from build123d import *

# Parameters (mm, degrees)
F0_W        = 40
F0_H        = 155
F1_DEPTH    = 3
F2_W        = 12.5
F2_H        = 13
F3_DEPTH    = 3
F4_R        = 8
F5_T1_DEPTH = 3
F6_R        = 1
F7_DEPTH    = 3
F8_DEPTH    = 15.3


# Not quite as in the source:
# - a fillet or chamfer that OpenCascade refuses, or shapes differently, is made with other operations: its cross-section is extruded or revolved along the edge and cut away or added


with BuildPart() as f1:
    # F0 (on Top) → F1 (new body)
    with BuildSketch(Plane.XY):
        Rectangle(F0_W, F0_H)
    extrude(amount=F1_DEPTH)

    # F2 (on face) → F3 (cut, through all)
    with BuildSketch(Plane.XY.offset(3)):
        with Locations((-13.75, -51)):
            Rectangle(F2_W, F2_H)
        with Locations((13.75, -51)):
            Rectangle(F2_W, F2_H)
    extrude(amount=-F3_DEPTH, mode=Mode.SUBTRACT)

    # F4
    f4_edges = [f1.edges().sort_by_distance(p)[0] for p in [
        (-20, -44.5, 1.5),
        (20, -44.5, 1.5),
        (20, -57.5, 1.5),
        (-20, -57.5, 1.5),
        (-20, -77.5, 1.5),
        (20, -77.5, 1.5),
        (-20, 77.5, 1.5),
        (20, 77.5, 1.5),
    ]]
    fillet(f4_edges, radius=F4_R)

    # F5: fillet of radius 7 on 4 edges, made by hand

    # F5_s2 → F5_t1 (join)
    with BuildSketch(Plane.XY):
        with BuildLine():
            ThreePointArc((-13.3333333333, -44.3881063775), (-9.1536616892, -46.7717188872), (-7.5, -51.2901994578))
            Line((-7.5, -51.2901994578), (-6.8, -51.2901994578))
            Line((-6.8, -51.2901994578), (-6.8, -44.5))
            Line((-6.8, -44.5), (-7.5, -43.8))
            ThreePointArc((-7.5, -43.8), (-12, -43.8), (-13.2166666667, -43.6978970694))
            Line((-13.2166666667, -43.6978970694), (-13.3333333333, -44.3881063775))
        make_face()
        with BuildLine():
            ThreePointArc((-7.5, -50.7098005422), (-9.1536616892, -55.2282811128), (-13.3333333333, -57.6118936225))
            Line((-13.3333333333, -57.6118936225), (-13.2166666667, -58.3021029306))
            ThreePointArc((-13.2166666667, -58.3021029306), (-12, -58.2), (-7.5, -58.2))
            Line((-7.5, -58.2), (-6.8, -57.5))
            Line((-6.8, -57.5), (-6.8, -50.7098005422))
            Line((-6.8, -50.7098005422), (-7.5, -50.7098005422))
        make_face()
        with BuildLine():
            ThreePointArc((13.3333333333, -44.3881063775), (9.1536616892, -46.7717188872), (7.5, -51.2901994578))
            Line((7.5, -51.2901994578), (6.8, -51.2901994578))
            Line((6.8, -51.2901994578), (6.8, -44.5))
            Line((6.8, -44.5), (7.5, -43.8))
            ThreePointArc((7.5, -43.8), (12, -43.8), (13.2166666667, -43.6978970694))
            Line((13.2166666667, -43.6978970694), (13.3333333333, -44.3881063775))
        make_face()
        with BuildLine():
            ThreePointArc((7.5, -50.7098005422), (9.1536616892, -55.2282811128), (13.3333333333, -57.6118936225))
            Line((13.3333333333, -57.6118936225), (13.2166666667, -58.3021029306))
            ThreePointArc((13.2166666667, -58.3021029306), (12, -58.2), (7.5, -58.2))
            Line((7.5, -58.2), (6.8, -57.5))
            Line((6.8, -57.5), (6.8, -50.7098005422))
            Line((6.8, -50.7098005422), (7.5, -50.7098005422))
        make_face()
    extrude(amount=F5_T1_DEPTH)

    # F6 (on face) → F7 (cut, through all)
    with BuildSketch(Plane.XY.offset(3)):
        with Locations((-15, -73.5)):
            Circle(F6_R)
        with Locations((-9, -73.5)):
            Circle(F6_R)
        with Locations((-3, -73.5)):
            Circle(F6_R)
        with Locations((3, -73.5)):
            Circle(F6_R)
        with Locations((-15, -28.8)):
            Circle(F6_R)
        with Locations((-9, -28.8)):
            Circle(F6_R)
        with Locations((-3, -28.8)):
            Circle(F6_R)
        with Locations((3, -28.8)):
            Circle(F6_R)
        with Locations((-15, 73.5)):
            Circle(F6_R)
        with Locations((-9, 73.5)):
            Circle(F6_R)
        with Locations((-3, 73.5)):
            Circle(F6_R)
        with Locations((3, 73.5)):
            Circle(F6_R)
        with Locations((9, -73.5)):
            Circle(F6_R)
        with Locations((15, -73.5)):
            Circle(F6_R)
        with Locations((9, -28.8)):
            Circle(F6_R)
        with Locations((15, -28.8)):
            Circle(F6_R)
        with Locations((9, 73.5)):
            Circle(F6_R)
        with Locations((15, 73.5)):
            Circle(F6_R)
    extrude(amount=-F7_DEPTH, mode=Mode.SUBTRACT)

    # F8 (add): a face of the model
    f8_faces = [f1.faces().sort_by_distance(p)[0] for p in [
        (0, 3.1365524685, 3),
    ]]
    extrude(f8_faces, amount=F8_DEPTH)


solid = f1.part
Could you check a few things on this model? Use its own coordinates, in mm. A direction names the side the tool comes from. Give positions to 0.01 mm unless a question says otherwise; leave off trailing zeros. Order: outer loops, then holes, each group sorted by start corner. A loop starts at its lowest first (then second) coordinate and runs counter-clockwise, first axis right, second up. Notation, with made-up numbers: (11, 25.5) -> (41, 25.5) arc R19 ccw to (41, 53.5) -> close; hole circle Ø8 at (20.5, -24). An arc over 180 degrees is marked (long way). Answer in a Markdown table with one row per item. Add a question column.
Item 1: We'd pull the mould along Y, two halves only. Please class faces 3 (the cylindrical face through (-9.205, -55.288, 9.022)), 4 (the flat face through (0, 1, 18.3)): pulls with the +Y half, pulls with the -Y half, needs draft (parallel to the pull), parting line crosses it, or undercut.
Item 2: Please list where these lines run through material, in increasing order: probe 1 along Y at (x, z) = (15, 4); probe 2 along Y at (x, z) = (-9, 13.25); probe 3 along X at (y, z) = (-70, 14).
Item 3: For faces 1 (the flat face through (-20, 16, 9)), 2 (the cylindrical face through (-9.293, -46.612, 9.022)), which set-ups out of +Z, -Z, +X, -X, +Y, -Y let a thin tool reach every point of the face, with its end or its side?
Item 4: I'm going to push flat-ended pins straight in: P1, Ø3, axis at x = 15, y = -58.5, coming from the -Z side; P2, Ø1.8, axis at x = 9, y = 73.5, coming from the +Z side. Where does each tip first touch, or does it pass through?
Item 5: Imagine slicing it at B-B (z = 15.25). Count the separate pieces of the cut face and the enclosed holes in it, and give its area (3 significant figures).
Item 6: Imagine slicing it at A-A (x = 17.5). List the corners of the cut face in (y, z) for me.
Result:
| question | item | result |
|---|---|---|
| 1 | face 3 | undercut |
| 1 | face 4 | needs draft |
| 2 | probe 1 | -76.92 to -74.5, -72.5 to -58.08, -43.92 to -29.8, -27.8 to 72.5, 74.5 to 76.92 |
| 2 | probe 2 | -77.5 to -74.5, -72.5 to -55.04, -46.96 to -29.8, -27.8 to 72.5, 74.5 to 77.5 |
| 2 | probe 3 | -19.98 to 19.98 |
| 3 | face 1 | +Z, -Z, -X, +Y, -Y |
| 3 | face 2 | +Z, -Z, -X |
| 4 | P1 | z = 0 |
| 4 | P2 | through |
| 5 | separate pieces | 1 |
| 5 | enclosed holes | 18 |
| 5 | area | 5,750 mm2 |
| 6 | outline | (-75.31, 0) -> (-59.69, 0) -> (-59.69, 18.3) -> (-75.31, 18.3) -> close; (-42.31, 0) -> (75.31, 0) -> (75.31, 18.3) -> (-42.31, 18.3) -> close |
